Build history of the part. All positions in model axes, mm. Face numbers are marked on the shaded views. A direction names the side the tool comes from. Coordinates: 2 decimals unless noted, no trailing zeros. Loops run counter-clockwise (first coordinate to the right, second up) from the corner with the lowest first, then second, coordinate; pieces in that order, holes last.
(1) Slice it at B-B (x = -21). Give the number of separate pieces and of enclosed holes in the cut face, and give its area (3 significant figures).
(2) Tool access for the marked faces 1, 2 and 3: list every direction of +Z, -Z, +X, -X, +Y, -Y with a clear straight run to the whole face (end or side of a thin tool).
(3) Wall check: L1, parallel to Y at x = -17, z = 25; L2, parallel to Y at x = -24, z = 0.5; L3, parallel to Z at x = 17.5, y = 17.5 (3 decimals). Give the ranges that are in metal, low to high.
(4) Slice it at A-A (y = 49). Give the cut face in (x, z) (3 decimals).
(5) Flat gauge pins, fed straight in: P1, Ø5, axis at x = -20.5, y = 46, coming from the +Z side; P2, Ø3, axis at y = 39, z = 2.5, coming from the -X side. Where does each tip first touch, or does it go through?
from build123d import *

# Parameters (mm, degrees)
SKETCH1_W           = 67.31
SKETCH1_H           = 67.31
SKETCH1_R           = 1.625
BOSS_EXTRUDE1_DEPTH = 8.89
BOSS_EXTRUDE2_DEPTH = 50.8
SKETCH3_R           = 2
CUT_EXTRUDE2_DEPTH  = 127


with BuildPart() as part:
    # Sketch1 → Boss-Extrude1 (new body)
    with BuildSketch(Plane(origin=(0, 0, 0), x_dir=(1, 0, 0), z_dir=(0, 1, 0))):
        Rectangle(SKETCH1_W, SKETCH1_H)
        with Locations(Location((17.960512242, 17.960512242, 0), (0, 0, 270))):
            Circle(SKETCH1_R, mode=Mode.SUBTRACT)
        with Locations(Location((-17.960512242, -17.960512242, 0), (0, 0, 270))):
            Circle(SKETCH1_R, mode=Mode.SUBTRACT)
    extrude(amount=BOSS_EXTRUDE1_DEPTH)

    # Sketch2 → Boss-Extrude2 (add)
    with BuildSketch(Plane(origin=(0, 8.89, 0), x_dir=(1, 0, 0), z_dir=(0, 1, 0))):
        Polygon((17.943087322, -33.655), (-33.655, 17.943087322), (-33.655, 5.370728753), (5.370728753, -33.655), align=None)
        Polygon((33.655, -17.943087322), (-17.943087322, 33.655), (-33.655, 33.655), (-33.655, 17.943087322), (17.943087322, -33.655), (33.655, -33.655), align=None)
        Polygon((-5.370728753, 33.655), (-17.943087322, 33.655), (33.655, -17.943087322), (33.655, -5.370728753), align=None)
    extrude(amount=BOSS_EXTRUDE2_DEPTH)

    # Sketch3 → Cut-Extrude2 (cut)
    with BuildSketch(Plane(origin=(-14.142135624, 0, 14.142135624), x_dir=(0.7071067811865464, 0, 0.7071067811865488), z_dir=(-0.7071067811865488, 0, 0.7071067811865464))):
        with Locations((-17.960512242, 52.250512242)):
            Circle(SKETCH3_R)
        with Locations((17.960512242, 16.329487758)):
            Circle(SKETCH3_R)
        with Locations((0, 34.29)):
            Circle(SKETCH3_R)
        with Locations((17.960512242, 52.250512242)):
            Circle(SKETCH3_R)
        with Locations((-17.960512242, 16.329487758)):
            Circle(SKETCH3_R)
    extrude(amount=-CUT_EXTRUDE2_DEPTH, mode=Mode.SUBTRACT)


solid = part.part
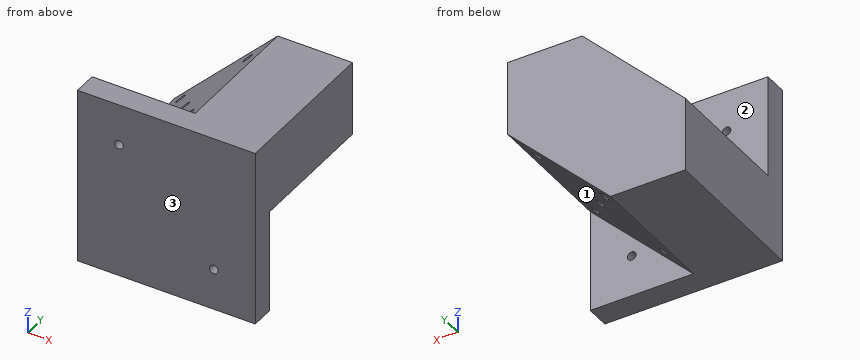
Response values:
1. separate pieces: 1
1. enclosed holes: 2
1. area: 2,640 mm2
2. face 1: -Z, +X, +Y
2. face 2: +Z, -X, +Y
2. face 3: +Z, -Z, +X, -X, -Y
3. L1: y = 0 to 8.89
3. L2: y = 0 to 14.85, 17.81 to 50.77, 53.73 to 59.69
3. L3: z = -10.784 to 5.607, 10.193 to 33.655
4. outline: (-33.655, -33.655) - (-5.371, -33.655) - (33.655, 5.371) - (33.655, 33.655) - (5.371, 33.655) - (-33.655, -5.371) - close
5. P1: stops at z = 10.28
5. P2: stops at x = -27.28
